The listing builds one solid part. Answer for the finished solid, in the listing's coordinates (mm). Give positions to 0.01 mm unless a question says otherwise; leave off trailing zeros. Loops run counter-clockwise (first coordinate to the right, second up) from the corner with the lowest first, then second, coordinate; pieces in that order, holes last. Notation, with made-up numbers: (36, 25) - (46, 25) arc R9 ccw to (46, 30) - close; hole circle Ø2 at (78, -34.5). An arc over 180 degrees is marked (long way). Write item = value, one per line. Start each with the question number.
1) Consider probe 1 along Y at (x, z) = (2.1, -24.25); probe 2 along Z at (x, y) = (2.2, -3); probe 3 along Y at (x, z) = (0.85, -12.5). Determine where each line is inside the solid, lowest interval first.
2) The part is cut by section D-D on x = 0.75. Write down the section's boundary in (y, z), plus the area to 3 significant figures.
3) The part is cut by section B-B on y = 10. Write down the section's boundary in (x, z).
4) The part is cut by section C-C on z = 24.25. Write down the section's boundary in (x, y).
5) The part is cut by section A-A on z = -8.5. Write down the section's boundary in (x, y).
from build123d import *

# Parameters (mm, degrees)
SKETCH1_W           = 80
SKETCH1_H           = 40
SKETCH1_R           = 2
SKETCH1_W_2         = 40
SKETCH1_H_2         = 20
BOSS_EXTRUDE1_DEPTH = 5
FILLET1_R           = 5


with BuildPart() as part:
    # Sketch1 → Boss-Extrude1 (new body)
    with BuildSketch(Plane(origin=(0, 0, 0), x_dir=(0, 0, -1), z_dir=(1, 0, 0))):
        Rectangle(SKETCH1_W, SKETCH1_H)
        with Locations((24.25, 10)):
            Circle(SKETCH1_R, mode=Mode.SUBTRACT)
        with Locations((24.25, 0)):
            Circle(SKETCH1_R, mode=Mode.SUBTRACT)
        with Locations(Location((-24.25, 10, 0), (0, 0, 180))):
            Circle(SKETCH1_R, mode=Mode.SUBTRACT)
        with Locations(Location((-24.25, 0, 0), (0, 0, 180))):
            Circle(SKETCH1_R, mode=Mode.SUBTRACT)
        with Locations((0, 5)):
            Rectangle(SKETCH1_W_2, SKETCH1_H_2, mode=Mode.SUBTRACT)
    extrude(amount=BOSS_EXTRUDE1_DEPTH)

    # Fillet1
    fillet1_edges = [part.edges().sort_by_distance(p)[0] for p in [
        (2.5, 20, 40),
        (2.5, 20, -40),
        (2.5, -20, -40),
        (2.5, -20, 40),
    ]]
    fillet(fillet1_edges, radius=FILLET1_R)


solid = part.part
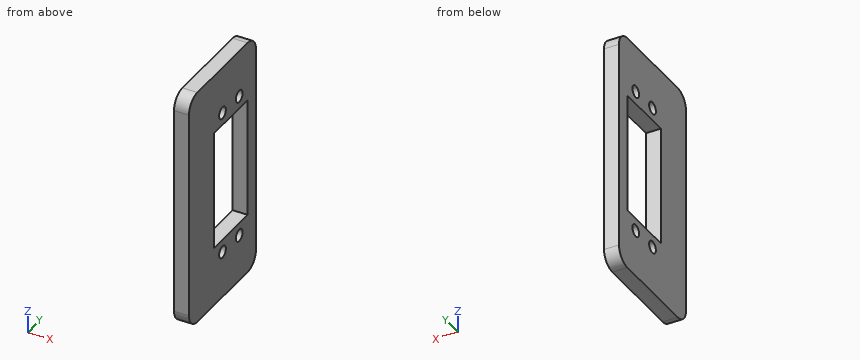
Answer below:
q1.probe_1 = -20 to -2, 2 to 8, 12 to 20
q1.probe_2 = -40 to -20, 20 to 40
q1.probe_3 = -20 to -5, 15 to 20
q2.outline = (-20, -35) arc R5 ccw to (-15, -40) - (15, -40) arc R5 ccw to (20, -35) - (20, 35) arc R5 ccw to (15, 40) - (-15, 40) arc R5 ccw to (-20, 35) - close; hole (-5, -20) - (15, -20) - (15, 20) - (-5, 20) - close; hole circle Ø4 at (0, -24.25); hole circle Ø4 at (0, 24.25); hole circle Ø4 at (10, -24.25); hole circle Ø4 at (10, 24.25)
q2.area = 2,330 mm2
q3.outline = (0, -40) - (5, -40) - (5, -26.25) - (0, -26.25) - close; (0, -22.25) - (5, -22.25) - (5, -20) - (0, -20) - close; (0, 20) - (5, 20) - (5, 22.25) - (0, 22.25) - close; (0, 26.25) - (5, 26.25) - (5, 40) - (0, 40) - close
q4.outline = (0, -20) - (5, -20) - (5, -2) - (0, -2) - close; (0, 2) - (5, 2) - (5, 8) - (0, 8) - close; (0, 12) - (5, 12) - (5, 20) - (0, 20) - close
q5.outline = (0, -20) - (5, -20) - (5, -5) - (0, -5) - close; (0, 15) - (5, 15) - (5, 20) - (0, 20) - close
